from build123d import *

# Parameters (mm, degrees)
BOSS_EXTRUDE1_DEPTH = 3.04


with BuildPart() as part:
    # Sketch1 → Boss-Extrude1 (new body)
    with BuildSketch(Plane(origin=(0, 0, 0), x_dir=(1, 0, 0), z_dir=(0, 1, 0))):
        with BuildLine():
            Line((0, 0), (60, 0))
            Line((60, 0), (60, 9.4))
            Line((60, 9.4), (53, 9.4))
            ThreePointArc((53, 9.4), (51.4, 11), (53, 12.6))
            Line((53, 12.6), (60, 12.6))
            Line((60, 12.6), (60, 22))
            Line((60, 22), (36, 22))
            Line((36, 22), (36, 11))
            ThreePointArc((36, 11), (30, 5), (24, 11))
            Line((24, 11), (24, 22))
            Line((24, 22), (0, 22))
            Line((0, 22), (0, 0))
        make_face()
        with BuildLine():
            Line((3.2, 12.6), (11.2, 12.6))
            ThreePointArc((11.2, 12.6), (12.8, 11), (11.2, 9.4))
            Line((11.2, 9.4), (3.2, 9.4))
            ThreePointArc((3.2, 9.4), (1.6, 11), (3.2, 12.6))
        make_face(mode=Mode.SUBTRACT)
    extrude(amount=BOSS_EXTRUDE1_DEPTH)


solid = part.part
CAD build for the part. Positions are in the model's coordinates, mm. A direction names the side the tool comes from. Coordinates: 2 decimals unless noted, no trailing zeros. Order: outer loops, then holes, each group sorted by start corner. A loop starts at its lowest first (then second) coordinate and runs counter-clockwise, first axis right, second up.
Item 1: Drill centre lines: L1, parallel to Z at x = 57, y = 1.95; L2, parallel to X at y = 1.35, z = -12; L3, parallel to X at y = 1.85, z = -13.5. Where is each one in solid material? Low to high.
Check sheet entries:
L1: z = -22 to -12.6, -9.4 to 0
L2: x = 0 to 1.95, 12.45 to 24, 36 to 51.75
L3: x = 0 to 24, 36 to 60
Item 2: Band-saw the part on B-B on z = -20. List the corners of the cut face in (x, y), plus the area to 3 significant figures.
Check sheet entries:
outline: (0, 0) - (24, 0) - (24, 3.04) - (0, 3.04) - close; (36, 0) - (60, 0) - (60, 3.04) - (36, 3.04) - close
area: 146 mm2
Item 3: Band-saw the part on D-D on x = 34. List the corners of the cut face in (y, z), plus the area to 3 significant figures.
Check sheet entries:
outline: (0, -6.53) - (3.04, -6.53) - (3.04, 0) - (0, 0) - close
area: 19.8 mm2
Item 4: 3-axis set-ups, long thin cutter, end or side, ignore diameter. For faces 1 (the face through (60, 1, -17)), 2 (the face through (1.6, 1.5, -11)), 3 (the face through (36, 1, -17)), 4 (the face through (56, 1, -12.6)), 5 (the face through (12, 1, -22)): which of +Z, -Z, +X, -X, +Y, -Y reach the whole face in a straight line?
Check sheet entries:
face 1: +Z, -Z, +X, +Y, -Y
face 2: +Y, -Y
face 3: -Z, +Y, -Y
face 4: +X, +Y, -Y
face 5: -Z, +X, -X, +Y, -Y
Item 5: Two-plate mould, pull along X, no slides. Class faces 6 (the face through (7, 1, -12.6)), 7 (the face through (0, 1, -11)), 8 (the face through (36.2, 0, -11.2)): +X half, -X half, draft (parallel to the pull), parting line (faces both ways), or undercut.
Check sheet entries:
face 6: undercut
face 7: -X half
face 8: draft
Item 6: Band-saw the part on A-A on x = 4. List the corners of the cut face in (y, z), plus the area to 3 significant figures.
Check sheet entries:
outline: (0, -22) - (3.04, -22) - (3.04, -12.6) - (0, -12.6) - close; (0, -9.4) - (3.04, -9.4) - (3.04, 0) - (0, 0) - close
area: 57.2 mm2
Item 7: Pin check, flat tips, straight feed: pin 1 Ø2 at (x, z) = (9, -17.5) entering from -Y; pin 2 Ø1 at (x, y) = (29.5, 2) entering from -Z. Stop position of each tip, or through.
Check sheet entries:
pin 1: stops at y = 0
pin 2: stops at z = -5.08
Item 8: Band-saw the part on C-C on y = 1.15. List the corners of the cut face in (x, z), plus the area to 3 significant figures.
Check sheet entries:
outline: (0, -22) - (24, -22) - (24, -11) arc R6 cw to (36, -11) - (36, -22) - (60, -22) - (60, -12.6) - (53, -12.6) arc R1.6 cw to (53, -9.4) - (60, -9.4) - (60, 0) - (0, 0) - close; hole (3.2, -12.6) - (11.2, -12.6) arc R1.6 ccw to (11.2, -9.4) - (3.2, -9.4) arc R1.6 ccw to start
area: 1,070 mm2
